Could you check a few things on this model? Use its own coordinates, in mm. A direction names the side the tool comes from. Give positions to 0.01 mm unless a question says otherwise; leave off trailing zeros. Write each loop counter-clockwise with the first axis right and the second up, starting at its lowest first coordinate (ties: lowest second). Pieces come first, ordered by that corner, then holes. Notation, with made-up numbers: (58.25, 4.5) - (77.25, 4.5) arc R23 ccw to (77.25, 16.5) - close; hole circle Ø11 at (80.25, 89.25). An arc over 180 degrees is marked (long way). Answer in a Markdown table with one row per item.
from build123d import *

# Parameters (mm, degrees)
SKETCH1_W           = 130
SKETCH1_H           = 175.5
BOSS_EXTRUDE1_DEPTH = 2
SKETCH2_W           = 29
SKETCH2_H           = 175.5
BOSS_EXTRUDE2_DEPTH = 2
SKETCH3_W           = 29
SKETCH3_H           = 175.5
BOSS_EXTRUDE3_DEPTH = 2
SKETCH4_W           = 10
SKETCH4_H           = 5
CUT_EXTRUDE1_DEPTH  = 4
FILLET1_R           = 20
FILLET2_R           = 1
SKETCH5_R           = 1.5
CUT_EXTRUDE2_DEPTH  = 2
SKETCH6_R           = 1.5
CUT_EXTRUDE3_DEPTH  = 2
SKETCH7_R           = 1.5
CUT_EXTRUDE4_DEPTH  = 2


with BuildPart() as part:
    # Sketch1 → Boss-Extrude1 (new body)
    with BuildSketch(Plane.XY):
        with Locations((65, 87.75)):
            Rectangle(SKETCH1_W, SKETCH1_H)
    extrude(amount=BOSS_EXTRUDE1_DEPTH)

    # Sketch2 → Boss-Extrude2 (add)
    with BuildSketch(Plane(origin=(130, 0, 0), x_dir=(0, 0, -1), z_dir=(1, 0, 0))):
        with Locations((-14.5, 87.75)):
            Rectangle(SKETCH2_W, SKETCH2_H)
    extrude(amount=BOSS_EXTRUDE2_DEPTH)

    # Sketch3 → Boss-Extrude3 (add)
    with BuildSketch(Plane.ZY):
        with Locations((14.5, 87.75)):
            Rectangle(SKETCH3_W, SKETCH3_H)
    extrude(amount=BOSS_EXTRUDE3_DEPTH)

    # Sketch4 → Cut-Extrude1 (cut)
    with BuildSketch(Plane.XY.offset(2)):
        with Locations((120.332257012, 2.5)):
            Rectangle(SKETCH4_W, SKETCH4_H)
    extrude(amount=-CUT_EXTRUDE1_DEPTH, mode=Mode.SUBTRACT)

    # Fillet1
    fillet1_edges = [part.edges().sort_by_distance(p)[0] for p in [
        (-1, 175.5, 29),
    ]]
    fillet(fillet1_edges, radius=FILLET1_R)

    # Fillet2
    fillet2_edges = [part.edges().sort_by_distance(p)[0] for p in [
        (115.332257012, 5, 1),
        (125.332257012, 5, 1),
    ]]
    fillet(fillet2_edges, radius=FILLET2_R)

    # Sketch5 → Cut-Extrude2 (cut)
    with BuildSketch(Plane.ZY.offset(-130)):
        with Locations((14.73, 167)):
            Circle(SKETCH5_R)
    extrude(amount=-CUT_EXTRUDE2_DEPTH, mode=Mode.SUBTRACT)

    # Sketch6 → Cut-Extrude3 (cut)
    with BuildSketch(Plane.XY.offset(2)):
        with Locations((113.75, 167)):
            Circle(SKETCH6_R)
    extrude(amount=-CUT_EXTRUDE3_DEPTH, mode=Mode.SUBTRACT)

    # Sketch7 → Cut-Extrude4 (cut)
    with BuildSketch(Plane(origin=(0, 0, 0), x_dir=(0, 0, -1), z_dir=(1, 0, 0))):
        with Locations((-10.5, 167)):
            Circle(SKETCH7_R)
    extrude(amount=-CUT_EXTRUDE4_DEPTH, mode=Mode.SUBTRACT)


solid = part.part
1) On a 3-axis mill with a long thin cutter (end or side, diameter ignored), from which of +Z, -Z, +X, -X, +Y, -Y can I reach the whole of each face in a straight line? I mean faces 1 (the face through (132, 89, 15)), 2 (the face through (130, 89, 16)). Say none if no direction works.
Check values:
| item | result |
|---|---|
| face 1 | +Z, -Z, +X, +Y, -Y |
| face 2 | +Z, +Y, -Y |
2) We'd pull the mould along Z, two halves only. Please class faces 3 (the face through (66, 87, 0)), 4 (the face through (130.2, 0, 11.1)), 5 (the face through (-1.014, 169.797, 22.986)): +Z half, -Z half, draft (parallel to the pull), parting line (faces both ways), or undercut.
Check values:
| item | result |
|---|---|
| face 3 | -Z half |
| face 4 | draft |
| face 5 | +Z half |
3) Imagine slicing it at C-C (x = 102). List the corners of the cut face in (y, z) for me, then the cut area to 3 significant figures.
Check values:
| item | result |
|---|---|
| outline | (0, 0) - (175.5, 0) - (175.5, 2) - (0, 2) - close |
| area | 351 mm2 |
4) Will these pins go through, and if not, where does the flat tip stop? P1, Ø12, axis at x = 65.5, z = 10.5, coming from the -Y side; P2, Ø2, axis at x = 119, z = 1, coming from the -Y side; P3, Ø5, axis at x = 42, y = 109, coming from the +Z side; P4, Ø2.5, axis at y = 167, z = 14.73, coming from the +X side.
Check values:
| item | result |
|---|---|
| P1 | passes through |
| P2 | stops at y = 5 |
| P3 | stops at z = 2 |
| P4 | stops at x = 0 |
5) Imagine slicing it at B-B (z = 25.75). List the corners of the cut face in (x, y) for me, then the cut area to 3 significant figures.
Check values:
| item | result |
|---|---|
| outline | (-2, 0) - (0, 0) - (0, 166.43) - (-2, 166.43) - close; (130, 0) - (132, 0) - (132, 175.5) - (130, 175.5) - close |
| area | 684 mm2 |
6) Imagine slicing it at A-A (y = 58.5). List the corners of the cut face in (x, z) for me, then the cut area to 3 significant figures.
Check values:
| item | result |
|---|---|
| outline | (-2, 0) - (132, 0) - (132, 29) - (130, 29) - (130, 2) - (0, 2) - (0, 29) - (-2, 29) - close |
| area | 376 mm2 |
7) If I drill on line 1 (Z direction, x = 130.4, y = 167); line 2 (Y direction, x = 113.75, z = 1.1); line 3 (X direction, y = 80, z = 26), over which ranges is the centre line in solid material (lowest first)?
Check values:
| item | result |
|---|---|
| line 1 | z = 0 to 13.23, 16.23 to 29 |
| line 2 | y = 0 to 165.5, 168.5 to 175.5 |
| line 3 | x = -2 to 0, 130 to 132 |
